from build123d import *

# Parameters (mm, degrees)
F2_SIZE2 = 10
F2_SIZE  = 7
F3_R     = 10
F4_SIZE  = 1


with BuildPart() as f1:
    # F0 (on Front) → F1 (revolve)
    with BuildSketch(Plane.XZ):
        Polygon((-69.8987477026, 18.6077695012), (-73.5294490392, 2), (-73.5294490392, 0), (39.3949043283, 0), (39.3949043283, 2), (10.4812397387, 10), (2.9812397387, 22.9903810568), (-11.0187602613, 22.9903810568), (-18.5187602613, 10), (-35.3987477026, 10), (-42.8987477026, 22.9903810568), align=None)
    revolve(axis=Axis((-13.5878343135, 0, -5), (1, 0, 0)))

    # F2
    f2_edges = [f1.edges().sort_by_distance(p)[0] for p in [
        (-69.898748, 0, -28.60777),
    ]]
    chamfer(f2_edges, length=F2_SIZE, length2=F2_SIZE2)

    # F3
    f3_edges = [f1.edges().sort_by_distance(p)[0] for p in [
        (-35.398748, 0, -20),
        (-18.51876, 0, -20),
        (10.48124, 0, -20),
        (-60.027938, 0, -30.209983),
        (2.98124, 0, -32.990381),
        (-71.393742, 0, -21.769272),
    ]]
    fillet(f3_edges, radius=F3_R)

    # F4
    f4_edges = [f1.edges().sort_by_distance(p)[0] for p in [
        (-73.529449, 0, -10),
        (39.394904, 0, -10),
    ]]
    chamfer(f4_edges, length=F4_SIZE)


solid = f1.part
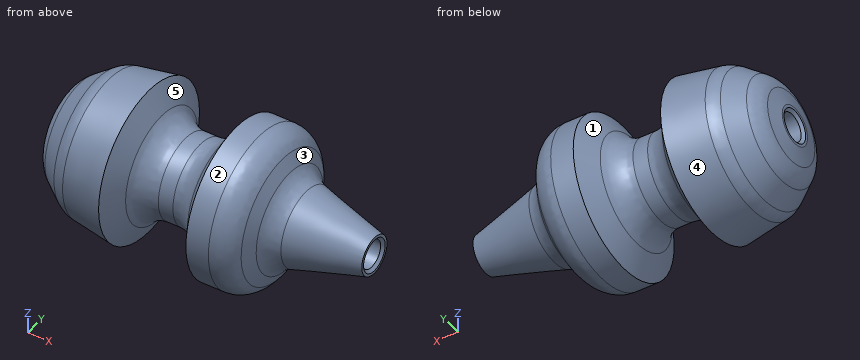
Can you work these out from the model? Positions are in its coordinate system, mm. Face numbers are marked on the shaded views. A direction names the side the tool comes from. Coordinates: 2 decimals unless noted, no trailing zeros. Order: outer loops, then holes, each group sorted by start corner. A loop starts at its lowest first (then second) coordinate and runs counter-clockwise, first axis right, second up. Notation, with made-up numbers: (70, 41) -> (103, 41) arc R24 cw to (103, 73) -> close; hole circle Ø7 at (83.25, 24). An arc over 180 degrees is marked (long way). Use one line per item in the form item = value.
Q1. I need wall thicknesses on L1, parallel to Z at x = -6, y = 0; L2, parallel to Y at x = -7, z = -5; L3, parallel to Z at x = -27, y = 0. Which ranges of each line are inside material? Lowest first, please.
From the geometry:
L1 = -32.99 to -10, 0 to 22.99
L2 = -27.99 to -5, 5 to 27.99
L3 = -20 to -10, 0 to 10
Q2. Will these pins go through, and if not, where does the flat tip stop? P1, Ø1, axis at y = -5, z = -23.5, coming from the +X side; P2, Ø8, axis at x = 21.5, y = 11, coming from the -Z side; P3, Ø3, axis at x = 3, y = 11, coming from the +Z side.
From the geometry:
P1 = 8.37
P2 = -14.99
P3 = 19.9
Q3. We'd pull the mould along X, two halves only. Please class the marked faces 3, 4 and 5: released by +X, released by -X, zero draft, split by the parting line, or undercut.
From the geometry:
face_3 = released by +X
face_4 = released by -X
face_5 = undercut
Q4. Imagine slicing it at A-A, the plane x = 27.5. List the corners of the cut face in (y, z) for me.
From the geometry:
outline = circle Ø20.58 at (0, -5); hole circle Ø10 at (0, -5)
Q5. Which directions (+Z, -Z, +X, -X, +Y, -Y) give clear straight access to the entire face, cutting with the end or side of a thin tool? Please do the marked faces 1 and 2.
From the geometry:
face_1 = none
face_2 = +X, -X
